from build123d import *

# Parameters (mm, degrees)
F0_R     = 9.8014094823
F0_R_2   = 5
F1_DEPTH = 50
F0_W     = 31.1324822545
F0_H     = 63.5031664371
F2_DEPTH = 25
F0_W_2   = 40
F0_H_2   = 4.5
F0_H_3   = 5.5
F3_DEPTH = 75
F4_R     = 9.99999
F5_DEPTH = 25


# Not quite as in the source:
# - a fillet or chamfer is up to 0.001 mm smaller than in the source, because OpenCascade refuses the exact size


with BuildPart() as f1:
    # F0 (on Top) → F1 (new body)
    with BuildSketch(Plane.XY):
        with Locations((-52.2364327669, -62.5)):
            Circle(F0_R)
        with Locations((-52.2364327669, -62.5)):
            Circle(F0_R_2, mode=Mode.SUBTRACT)
    extrude(amount=F1_DEPTH)



with BuildPart() as f1b:
    # F0 (on Top) → F1, piece 2 (new body)
    with BuildSketch(Plane.XY):
        with Locations((-52.2364327669, 62.5)):
            Circle(F0_R)
        with Locations((-52.2364327669, 62.5)):
            Circle(F0_R_2, mode=Mode.SUBTRACT)
    extrude(amount=F1_DEPTH)


with BuildPart() as f1_1:
    add(f1.part)

    add(f1b.part)  # F2 merges F1b
    # F0 (on Top) → F2 (join)
    with BuildSketch(Plane.XY):
        with Locations((-52.1973261058, 41.7515832186)):
            Rectangle(F0_W, F0_H)
        with Locations((-52.2364327669, 62.5)):
            Circle(F0_R, mode=Mode.SUBTRACT)
        Polygon((-36.6310849786, -10), (27.7635672331, -10), (27.7635672331, -5.5), (27.7635672331, 0), (27.7635672331, 5.5), (27.7635672331, 10), (-36.6310849786, 10), (-67.7635672331, 10), (-67.7635672331, -10), align=None)
        with Locations((-52.1973261058, -41.7515832186)):
            Rectangle(F0_W, F0_H)
        with Locations((-52.2364327669, -62.5)):
            Circle(F0_R, mode=Mode.SUBTRACT)
    extrude(amount=F2_DEPTH)

    # F0 (on Top) → F3 (join)
    with BuildSketch(Plane.XY):
        with Locations((47.7635672331, -7.75)):
            Rectangle(F0_W_2, F0_H_2)
        with Locations((47.7635672331, -2.75)):
            Rectangle(F0_W_2, F0_H_3)
        with Locations((47.7635672331, 2.75)):
            Rectangle(F0_W_2, F0_H_3)
        with Locations((47.7635672331, 7.75)):
            Rectangle(F0_W_2, F0_H_2)
    extrude(amount=F3_DEPTH)

    # F4 (radius 10 in the source; OpenCascade refuses exactly that, so slightly less here)
    f4_edges = [f1_1.edges().sort_by_distance(p)[0] for p in [
        (47.763567, -10, 75),
        (67.763567, 0, 75),
        (47.763567, 10, 75),
        (27.763567, 0, 75),
    ]]
    fillet(f4_edges, radius=F4_R)

    # F0 (on Top) → F5 (join)
    with BuildSketch(Plane.XY):
        with Locations((-52.2364327669, 62.5)):
            Circle(F0_R_2)
        with Locations((-52.2364327669, -62.5)):
            Circle(F0_R_2)
    extrude(amount=F5_DEPTH)


solid = f1_1.part
Geometry check sheet. Reference: the model listing, model coordinates, mm. A direction names the side the tool comes from. Give positions to 0.01 mm unless a question says otherwise; leave off trailing zeros. Loops run counter-clockwise (first coordinate to the right, second up) from the corner with the lowest first, then second, coordinate; pieces in that order, holes last. Notation, with made-up numbers: M 83.25,62.5 L 121.25,62.5 A18 ccw 121.25,76.5 Z; hole C 34.25,-25 d9. An arc over 180 degrees is marked long. Answer as a JSON object with one key per item and string values. Group by question number.
Item 1: Material ranges on L1, parallel to X at y = 62, z = 35; L2, parallel to Y at x = -56.5, z = 45.5; L3, parallel to Z at x = -48.5, y = 16, recorded low to high.
Item 2: Sectioned sample at C-C on x = 3. Record the boundary of the cut face in (y, z).
Item 3: Sectioned sample at A-A on y = 62.5. Record the boundary of the cut face in (x, z).
Item 4: Sectioned sample at B-B on z = 7. Record the boundary of the cut face in (x, y), plus the area to 3 significant figures.
Item 5: Access from +Z, -Z, +X, -X, +Y, -Y to the whole of each face (thin tool, end or side, straight path). Record for faces 1 (the flat face through (-52, 63, 25)), 2 (the flat face through (26.4, -10, 24.8)), 3 (the flat face through (27.764, 0, 45)), 4 (the flat face through (-36.631, 41, 12)).
Item 6: Mould release check, pull along Y, two halves, no side actions. Record for faces 5 (the flat face through (67.764, 0, 32)), 6 (the flat face through (-42, 1, 25)), 7 (the flat face through (-52, -73.503, 12)), 8 (the flat face through (-52, 73.503, 12)): pulls with the +Y half, pulls with the -Y half, needs draft (parallel to the pull), parting line crosses it, or undercut.
Item 7: Sectioned sample at D-D on y = -2. Record the boundary of the cut face in (x, z), plus the area to 3 significant figures.
Item 8: Gauge pin test, flat ends, axial feed: pin 1 (21.5 mm diameter, centred on x = -53, y = -66.5, fed in from +Z); pin 2 (10 mm diameter, centred on x = 32.5, z = 40, fed in from +Y); pin 3 (10 mm diameter, centred on x = 36, z = 49.5, fed in from -Y); pin 4 (9 mm diameter, centred on x = -52.24, y = 62.5, fed in from -Z). Record the tip position at first contact, or that the pin passes through.
Findings below:
{
 "1": {"L1": "-62.03 to -57.21, -47.26 to -42.45", "L2": "-71.33 to -65.11, -59.89 to -53.67, 53.67 to 59.89, 65.11 to 71.33", "L3": "0 to 25"},
 "2": {"outline": "M -10,0 L 10,0 L 10,25 L -10,25 Z"},
 "3": {"outline": "M -67.76,0 L -36.63,0 L -36.63,25 L -42.44,25 L -42.44,50 L -47.24,50 L -47.24,25 L -57.24,25 L -57.24,50 L -62.04,50 L -62.04,25 L -67.76,25 Z"},
 "4": {"outline": "M -67.76,-73.5 L -36.63,-73.5 L -36.63,-10 L 67.76,-10 L 67.76,10 L -36.63,10 L -36.63,73.5 L -67.76,73.5 Z", "area": "6,660 mm2"},
 "5": {"face 1": "+Z", "face 2": "+Z, -Z, +X, -Y", "face 3": "+Z, -X, +Y, -Y", "face 4": "+Z, -Z, +X, +Y"},
 "6": {"face 5": "needs draft", "face 6": "undercut", "face 7": "pulls with the -Y half", "face 8": "pulls with the +Y half"},
 "7": {"outline": "M -67.76,0 L 67.76,0 L 67.76,65 A10 ccw 59.76,74.8 L 35.76,74.8 A10 ccw 27.76,65 L 27.76,25 L -67.76,25 Z", "area": "5,340 mm2"},
 "8": {"pin 1": "z = 50", "pin 2": "y = 10", "pin 3": "y = -10", "pin 4": "z = 0"}
}
